Input: dimensioned drawing with shaded views. Units: mm. Origin: part minimum x, y, z. Give positions to 0.01 mm unless a question says otherwise; leave off trailing zeros. Loops run counter-clockwise (first coordinate to the right, second up) from the corner with the lowest first, then second, coordinate; pieces in that order, holes last. Notation, with made-up numbers: (40.5, 16.25) -> (81.5, 16.25) arc R4 ccw to (81.5, 21.25) -> close; hole circle Ø7 at (-9.75, 71.5). An arc over 180 degrees is marked (long way). One line per question, with ' | ' between items. Start each with the question number.
Item 1: Section A-A on x = 428.5. Return loops of the section in (y, z).
Item 2: Section D-D on z = 307.5. Return loops of the section in (x, y).
Item 3: Section C-C on z = 200. Return loops of the section in (x, y), then the cut area to 3 significant figures.
Item 4: Pin query (flat end, axial travel): P1, Ø3.5, axis at y = 8.5, z = 149, coming from the -X side; P2, Ø6, axis at x = 164.5, z = 220.5, coming from the -Y side; P3, Ø16, axis at y = 18, z = 262, coming from the +X side. Return the tip coordinate at first contact, or that it passes through.
Item 5: Section B-B on y = 23. Return loops of the section in (x, z).
Item 6: Mould query, pull axis X, two halves, no side actions, for the marked faces 1, 2 and 3. Classes: released by +X, released by -X, zero draft, split by the parting line, or undercut.
Item 7: Material intervals for line 1 along X through (y, z) = (104, 200); line 2 along X through (y, z) = (14.5, 25.5); line 3 along Z through (x, y) = (250, 77), sorted ascending. Write a range as [from, to].
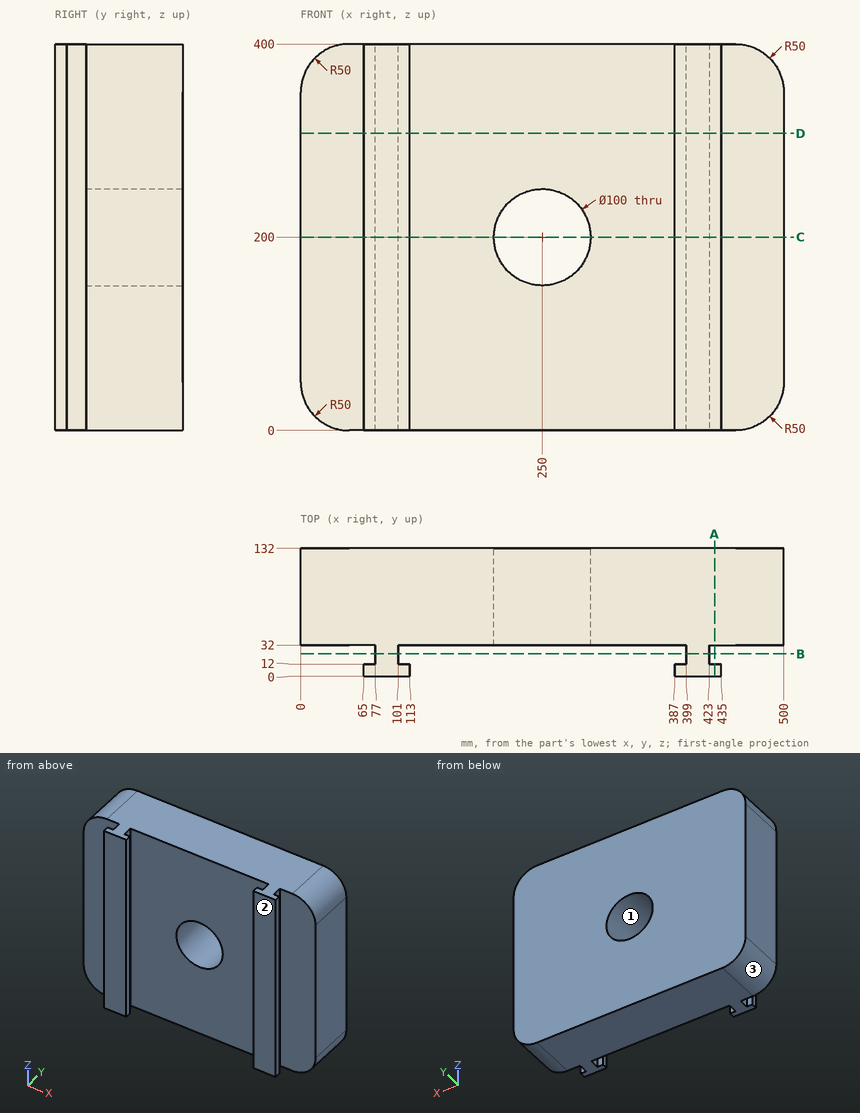
Result sheet:
1) outline: (0, 0) -> (12, 0) -> (12, 400) -> (0, 400) -> close; (32, 0) -> (132, 0) -> (132, 400) -> (32, 400) -> close
2) outline: (0, 32) -> (77, 32) -> (77, 12) -> (65, 12) -> (65, 0) -> (113, 0) -> (113, 12) -> (101, 12) -> (101, 32) -> (399, 32) -> (399, 12) -> (387, 12) -> (387, 0) -> (435, 0) -> (435, 12) -> (423, 12) -> (423, 32) -> (500, 32) -> (500, 132) -> (0, 132) -> close
3) outline: (0, 32) -> (77, 32) -> (77, 12) -> (65, 12) -> (65, 0) -> (113, 0) -> (113, 12) -> (101, 12) -> (101, 32) -> (200, 32) -> (200, 132) -> (0, 132) -> close; (300, 32) -> (399, 32) -> (399, 12) -> (387, 12) -> (387, 0) -> (435, 0) -> (435, 12) -> (423, 12) -> (423, 32) -> (500, 32) -> (500, 132) -> (300, 132) -> close | area: 42,100 mm²
4) P1: stops at x = 65 | P2: stops at y = 32 | P3: stops at x = 435
5) outline: (77, 0) -> (101, 0) -> (101, 400) -> (77, 400) -> close; (399, 0) -> (423, 0) -> (423, 400) -> (399, 400) -> close
6) face 1: undercut | face 2: zero draft | face 3: released by -X
7) line 1: x = [0, 200], [300, 500] | line 2: x = [77, 101], [399, 423] | line 3: z = [0, 150], [250, 400]
